Can you work these out from the model? Positions are in its coordinate system, mm. Face numbers are marked on the shaded views. Coordinates: 2 decimals unless noted, no trailing zeros. Order: outer loops, then holes, each group sorted by start corner. A loop starts at its lowest first (then second) coordinate and runs counter-clockwise, first axis right, second up. Notation, with made-up numbers: (61, 79.5) -> (87, 79.5) arc R14 ccw to (87, 105.5) -> close; hole circle Ø1 at (86, -11). An arc over 180 degrees is marked (long way). Answer as CSV lines item,"result".
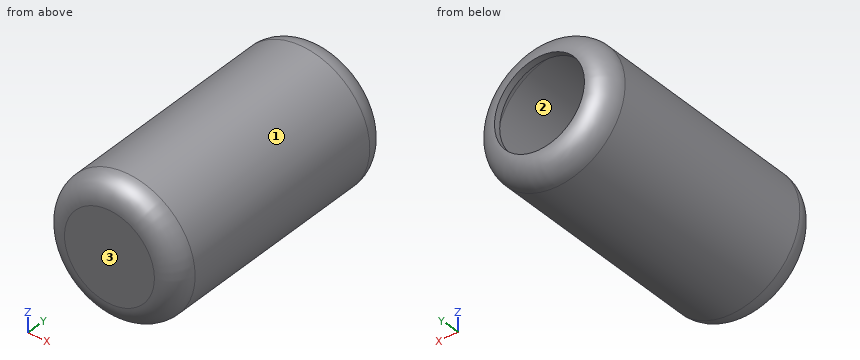
from build123d import *

# Parameters (mm, degrees)
SKETCH1_R           = 10.5
BOSS_EXTRUDE1_DEPTH = 40.5
FILLET1_R           = 3.5


# Read off the part's stored shape, not the designer's step: Shell4
with BuildPart() as part:
    # Sketch1 → Boss-Extrude1 (new body)
    with BuildSketch(Plane(origin=(0, 0, 0), x_dir=(1, 0, 0), z_dir=(0, 1, 0))):
        with Locations(Location((0, 0, 0), (0, 0, 270))):
            Circle(SKETCH1_R)
    extrude(amount=BOSS_EXTRUDE1_DEPTH)

    # Fillet1
    fillet1_edges = [part.edges().sort_by_distance(p)[0] for p in [
        (0, 0, -10.5),
        (0, 40.5, -10.5),
    ]]
    fillet(fillet1_edges, radius=FILLET1_R)

    # Shell4 outline → Shell4 (revolve, cut)
    with BuildSketch(Plane.XY):
        with BuildLine():
            Line((0, 1), (7, 1))
            ThreePointArc((7, 1), (8.767766953, 1.732233047), (9.5, 3.5))
            Line((9.5, 3.5), (9.5, 37))
            ThreePointArc((9.5, 37), (8.767766953, 38.767766953), (7, 39.5))
            Line((7, 39.5), (7, 40.5))
            Line((7, 40.5), (0, 40.5))
            Line((0, 40.5), (0, 1))
        make_face()
    revolve(axis=Axis((0, 0, 0), (0, 1, 0)), mode=Mode.SUBTRACT)


solid = part.part
Q1. We'd pull the mould along Z, two halves only. Please class the marked faces 1, 2 and 3: pulls with the +Z half, pulls with the -Z half, needs draft (parallel to the pull), parting line crosses it, or undercut.
Solution:
face 1,"parting line crosses it"
face 2,"undercut"
face 3,"needs draft"
Q2. If I drill on line 1 (Z direction, x = 0.25, y = 22); line 2 (Z direction, x = 7.25, y = 11), over which ranges is the centre line in solid material (lowest first)?
Solution:
line 1,"-10.5 to -9.5, 9.5 to 10.5"
line 2,"-7.6 to -6.14, 6.14 to 7.6"
Q3. Imagine slicing it at B-B (x = 0). List the corners of the cut face in (y, z) for me.
Solution:
outline,"(0, -7) arc R3.5 ccw to (3.5, -10.5) -> (37, -10.5) arc R3.5 ccw to (40.5, -7) -> (39.5, -7) arc R2.5 cw to (37, -9.5) -> (3.5, -9.5) arc R2.5 cw to (1, -7) -> (1, 7) arc R2.5 cw to (3.5, 9.5) -> (37, 9.5) arc R2.5 cw to (39.5, 7) -> (40.5, 7) arc R3.5 ccw to (37, 10.5) -> (3.5, 10.5) arc R3.5 ccw to (0, 7) -> close"
Q4. Imagine slicing it at D-D (y = 38). List the corners of the cut face in (x, z) for me.
Solution:
outline,"circle Ø20.71 at (0, 0); hole circle Ø18.58 at (0, 0)"
Q5. Imagine slicing it at A-A (z = 0). List the corners of the cut face in (x, y) for me, and give its area (3 significant figures).
Solution:
outline,"(-10.5, 3.5) arc R3.5 ccw to (-7, 0) -> (7, 0) arc R3.5 ccw to (10.5, 3.5) -> (10.5, 37) arc R3.5 ccw to (7, 40.5) -> (7, 39.5) arc R2.5 cw to (9.5, 37) -> (9.5, 3.5) arc R2.5 cw to (7, 1) -> (-7, 1) arc R2.5 cw to (-9.5, 3.5) -> (-9.5, 37) arc R2.5 cw to (-7, 39.5) -> (-7, 40.5) arc R3.5 ccw to (-10.5, 37) -> close"
area,"99.8 mm2"
Q6. For P1, Ø11, axis at x = 2.5, z = -2.5, coming from the +Y side; P2, Ø1.5, axis at x = -5, y = 28, coming from the +Z side; P3, Ø6, axis at x = 2, z = 2, coming from the +Y side; P4, Ø8, axis at y = 12, z = 7, coming from the -X side, each with a flat end and sliding along its axis, tell me the tip position at first contact or that it passes through.
Solution:
P1,"y = 40.5"
P2,"z = 9.6"
P3,"y = 1"
P4,"x = -10.06"
Q7. Imagine slicing it at C-C (y = 27). List the corners of the cut face in (x, z) for me.
Solution:
outline,"circle Ø21 at (0, 0); hole circle Ø19 at (0, 0)"
